from build123d import *

# Parameters (mm, degrees)
F0_W     = 609.6
F0_H     = 133.35
F1_DEPTH = 5.9944
F2_R     = 4.7625
F3_DEPTH = 11.9888


with BuildPart() as f1:
    # F0 (on Right) → F1 (new body, symmetric)
    with BuildSketch(Plane.YZ):
        Rectangle(F0_W, F0_H)
    extrude(amount=F1_DEPTH, both=True)

    # F2 (on face) → F3 (cut, through all)
    with BuildSketch(Plane.YZ.offset(5.9944)):
        with Locations((-238.125, -44.45)):
            Circle(F2_R)
        with Locations((-47.625, -44.45)):
            Circle(F2_R)
        with Locations((-47.625, 44.45)):
            Circle(F2_R)
        with Locations((-238.125, 44.45)):
            Circle(F2_R)
    extrude(amount=-F3_DEPTH, mode=Mode.SUBTRACT)


solid = f1.part
Input: part model. Units: mm. Frame: model coordinates. Round coordinates to 2 decimals unless told otherwise and drop trailing zeros.
1) Ray query, L1, parallel to Y at x = 0.5, z = -45.5; L2, parallel to Y at x = -5, z = 43; L3, parallel to Z at x = 2, y = -234.5 (3 decimals). Return the intervals inside material, ascending.
2) Contact query for a flat-ended pin moving along its axis: P1, Ø5.5, axis at y = -238.125, z = -44.45, coming from the -X side. Output: stop coordinate, or through.
3) Draft query along Z for faces 1 (the flat face through (0, -4, 66.675)), 2 (the cylindrical face through (0.084, -45.065, -40.434)), 3 (the cylindrical face through (0.084, -45.427, 40.225)), 4 (the flat face through (0, 304.8, -1)). Return one class per face: pulls with the +Z half, pulls with the -Z half, needs draft (parallel to the pull), parting line crosses it, or undercut.
Geometry says:
1. L1: y = -304.8 to -242.77, -233.48 to -52.27, -42.98 to 304.8
1. L2: y = -304.8 to -242.66, -233.59 to -52.16, -43.09 to 304.8
1. L3: z = -66.675 to -47.539, -41.361 to 41.361, 47.539 to 66.675
2. P1: passes through
3. face 1: pulls with the +Z half
3. face 2: undercut
3. face 3: undercut
3. face 4: needs draft
